Geometry: final body of the model. Coordinates: model frame, mm. Face numbers are marked on the shaded views. A direction names the side the tool comes from. Round coordinates to 2 decimals unless told otherwise and drop trailing zeros. Order: outer loops, then holes, each group sorted by start corner. A loop starts at its lowest first (then second) coordinate and runs counter-clockwise, first axis right, second up. Notation, with made-up numbers: (82, 29) -> (113, 29) arc R32 ccw to (113, 56) -> close; hole circle Ø11 at (80, -39). An arc over 180 degrees is marked (long way). Put each result on its own line as item: value.
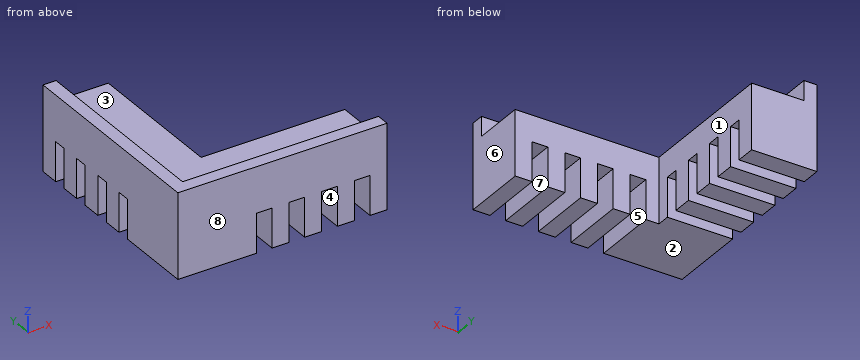
```python
from build123d import *

# Parameters (mm, degrees)
F1_DEPTH = 13
F0_W     = 8
F0_H     = 22
F2_DEPTH = 10
F3_W     = 2.409125
F3_H     = 6
F5_DEPTH = 25
F4_W     = 2
F4_H     = 6
F6_DEPTH = 25


with BuildPart() as f1:
    # F0 (on Top) → F1 (new body)
    with BuildSketch(Plane.XY):
        Polygon((0, -8), (0, 0), (0, 22), (-2, 22), (-2, 11.907217), (-2, -10), (30, -10), (30, -8), align=None)
    extrude(amount=F1_DEPTH)

    # F0 (on Top) → F2 (join)
    with BuildSketch(Plane.XY):
        with Locations((4, 11)):
            Rectangle(F0_W, F0_H)
        Polygon((8, 0), (0, 0), (0, -8), (30, -8), (30, 0), align=None)
    extrude(amount=F2_DEPTH)

    # F3 (on face) → F5 (cut)
    with BuildSketch(Plane.XZ.offset(10)):
        with Locations((11.204562, 3)):
            Rectangle(F3_W, F3_H)
        with Locations((16.204563, 3)):
            Rectangle(F3_W, F3_H)
        with Locations((21.204563, 3)):
            Rectangle(F3_W, F3_H)
        with Locations((26.204563, 3)):
            Rectangle(F3_W, F3_H)
    extrude(amount=-F5_DEPTH, mode=Mode.SUBTRACT)

    # F4 (on face) → F6 (cut)
    with BuildSketch(Plane(origin=(-2, 0, 0), x_dir=(0, -1, 0), z_dir=(-1, 0, 0))):
        with Locations((-13, 3)):
            Rectangle(F4_W, F4_H)
        with Locations((-18, 3)):
            Rectangle(F4_W, F4_H)
        with Locations((-8, 3)):
            Rectangle(F4_W, F4_H)
        with Locations((-3, 3)):
            Rectangle(F4_W, F4_H)
    extrude(amount=-F6_DEPTH, mode=Mode.SUBTRACT)


solid = f1.part
```
1. Cut plane D-D on z = 4.5. State how many separate pieces and enclosed holes the cut face has, and give its area (3 significant figures).
Ans:
separate pieces: 9
enclosed holes: 0
area: 364 mm²
2. Material intervals for probe 1 along X at (y, z) = (-2, 4.5); probe 2 along Y at (x, z) = (1, 5); probe 3 along Y at (x, z) = (15, 10.5), sorted ascending.
Ans:
probe 1: -2 to 10, 12.41 to 15, 17.41 to 20, 22.41 to 25, 27.41 to 30
probe 2: -10 to 2, 4 to 7, 9 to 12, 14 to 17, 19 to 22
probe 3: -10 to -8
3. Set-up query: the marked faces 1, 2, 3 and 4. Return all of +Z, -Z, +X, -X, +Y, -Y with unobstructed straight access to the full face (end or side cutting, diameter ignored); none if empty.
Ans:
face 1: +Z, -Z, +X, +Y
face 2: -Z, +X, -X, +Y, -Y
face 3: +Z, +X, +Y
face 4: -Z, +Y, -Y
4. Contact query for flat-ended pins moving along their axis: P1, Ø0.6, axis at x = 4, y = 2.5, coming from the -Z side; P2, Ø1, axis at x = 9.5, z = 9, coming from the +Y side; P3, Ø2, axis at x = 5, y = 0.5, coming from the -Z side; P4, Ø2.5, axis at x = 15.5, z = 11.5, coming from the +Y side. Output: stop coordinate, or through.
Ans:
P1: z = 6
P2: y = 0
P3: z = 0
P4: y = -8
5. Cut plane C-C on z = 11.5. Return loops of the section in (x, y), and give its area (3 significant figures).
Ans:
outline: (-2, -10) -> (30, -10) -> (30, -8) -> (0, -8) -> (0, 22) -> (-2, 22) -> close
area: 124 mm²
6. Cut plane B-B on x = 11.5. Return loops of the section in (y, z), and give its area (3 significant figures).
Ans:
outline: (-10, 6) -> (0, 6) -> (0, 10) -> (-8, 10) -> (-8, 13) -> (-10, 13) -> close
area: 46.0 mm²
7. Cut plane A-A on y = -5. Return loops of the section in (x, z), and give its area (3 significant figures).
Ans:
outline: (-2, 0) -> (10, 0) -> (10, 6) -> (12.41, 6) -> (12.41, 0) -> (15, 0) -> (15, 6) -> (17.41, 6) -> (17.41, 0) -> (20, 0) -> (20, 6) -> (22.41, 6) -> (22.41, 0) -> (25, 0) -> (25, 6) -> (27.41, 6) -> (27.41, 0) -> (30, 0) -> (30, 10) -> (0, 10) -> (0, 13) -> (-2, 13) -> close
area: 268 mm²
8. Draft query along X for the marked faces 5, 6, 7 and 8. Return one class per face: +X half, -X half, draft (parallel to the pull), parting line (faces both ways), or undercut.
Ans:
face 5: undercut
face 6: +X half
face 7: undercut
face 8: draft
